from build123d import *

# Parameters (mm, degrees)
SKETCH1_W               = 101.6
SKETCH1_H               = 76.2
BOSS_EXTRUDE1_DEPTH     = 177.8
SHELL1_T                = -5.08
SKETCH2_W               = 2.667
SKETCH2_H               = 2.667
CUT_EXTRUDE1_DEPTH      = 15.24
CUT_EXTRUDE1_DRAFT      = -1
MIRROR1_COPY_1_SKETCH_W = 2.667
MIRROR1_COPY_1_SKETCH_H = 2.667
MIRROR1_COPY_1_DEPTH    = 15.24
MIRROR1_COPY_1_DRAFT    = -1
MIRROR2_COPY_1_SKETCH_W = 2.667
MIRROR2_COPY_1_SKETCH_H = 2.667
MIRROR2_COPY_1_DEPTH    = 15.24
MIRROR2_COPY_1_DRAFT    = -1
MIRROR2_COPY_2_SKETCH_W = 2.667
MIRROR2_COPY_2_SKETCH_H = 2.667
MIRROR2_COPY_2_DEPTH    = 15.24
MIRROR2_COPY_2_DRAFT    = -1
MIRROR3_COPY_1_SKETCH_W = 2.667
MIRROR3_COPY_1_SKETCH_H = 2.667
MIRROR3_COPY_1_DEPTH    = 15.24
MIRROR3_COPY_1_DRAFT    = -1
MIRROR3_COPY_2_SKETCH_W = 2.667
MIRROR3_COPY_2_SKETCH_H = 2.667
MIRROR3_COPY_2_DEPTH    = 15.24
MIRROR3_COPY_2_DRAFT    = -1
MIRROR3_COPY_3_SKETCH_W = 2.667
MIRROR3_COPY_3_SKETCH_H = 2.667
MIRROR3_COPY_3_DEPTH    = 15.24
MIRROR3_COPY_3_DRAFT    = -1
MIRROR3_COPY_4_SKETCH_W = 2.667
MIRROR3_COPY_4_SKETCH_H = 2.667
MIRROR3_COPY_4_DEPTH    = 15.24
MIRROR3_COPY_4_DRAFT    = -1
SKETCH3_W               = 63.5
SKETCH3_H               = 91.44
SKETCH3_W_2             = 58.42
SKETCH3_H_2             = 86.36
EXTRUDE_THIN1_DEPTH     = 12.7
SKETCH4_W               = 25.4
SKETCH4_H               = 91.44
CUT_EXTRUDE_THIN1_DEPTH = 12.7
FILLET1_R               = 2.54


with BuildPart() as part:
    # Sketch1 → Boss-Extrude1 (new body)
    with BuildSketch(Plane(origin=(0, 0, 0), x_dir=(1, 0, 0), z_dir=(0, 1, 0))):
        Rectangle(SKETCH1_W, SKETCH1_H)
    extrude(amount=BOSS_EXTRUDE1_DEPTH)

    # Shell1
    shell1_openings = [part.faces().sort_by_distance(p)[0] for p in [
        (0, 177.8, 0),
        (0, 0, 0),
    ]]
    offset(amount=SHELL1_T, openings=shell1_openings, kind=Kind.INTERSECTION)


with BuildPart() as cut_extrude1_tool:
    # Sketch2 → Cut-Extrude1 (with draft: the straight prism first)
    with BuildSketch(Plane(origin=(0, 177.8, 0), x_dir=(1, 0, 0), z_dir=(0, 1, 0))):
        with Locations((-48.26, 35.56)):
            Rectangle(SKETCH2_W, SKETCH2_H)
    extrude(amount=-CUT_EXTRUDE1_DEPTH)
    # Cut-Extrude1: the draft: its side faces are tilted about the plane it starts from
    cut_extrude1_sides = [cut_extrude1_tool.faces().sort_by_distance(p)[0] for p in [
        (-49.5935, 170.18, -35.56),
        (-48.26, 170.18, -34.2265),
        (-46.9265, 170.18, -35.56),
        (-48.26, 170.18, -36.8935),
    ]]
    draft(cut_extrude1_sides, Plane(origin=(0, 177.8, 0), x_dir=(1, 0, 0), z_dir=(0, 1, 0)), CUT_EXTRUDE1_DRAFT)


with BuildPart() as part_1:
    add(part.part)

    # Cut-Extrude1: cut by cut_extrude1_tool
    add(cut_extrude1_tool.part, mode=Mode.SUBTRACT)


with BuildPart() as mirror1_copy_1_tool:
    # Mirror1 copy 1 sketch → Mirror1 copy 1 (with draft: the straight prism first)
    with BuildSketch(Plane(origin=(0, 177.8, 0), x_dir=(1, 0, 0), z_dir=(0, 1, 0))):
        with Locations((-48.26, -35.56)):
            Rectangle(MIRROR1_COPY_1_SKETCH_W, MIRROR1_COPY_1_SKETCH_H)
    extrude(amount=-MIRROR1_COPY_1_DEPTH)
    # Mirror1 copy 1: the draft: its side faces are tilted about the plane it starts from
    mirror1_copy_1_sides = [mirror1_copy_1_tool.faces().sort_by_distance(p)[0] for p in [
        (-49.5935, 170.18, 35.56),
        (-48.26, 170.18, 34.2265),
        (-46.9265, 170.18, 35.56),
        (-48.26, 170.18, 36.8935),
    ]]
    draft(mirror1_copy_1_sides, Plane(origin=(0, 177.8, 0), x_dir=(1, 0, 0), z_dir=(0, 1, 0)), MIRROR1_COPY_1_DRAFT)


with BuildPart() as part_2:
    add(part_1.part)

    # Mirror1 copy 1: cut by mirror1_copy_1_tool
    add(mirror1_copy_1_tool.part, mode=Mode.SUBTRACT)


with BuildPart() as mirror2_copy_1_tool:
    # Mirror2 copy 1 sketch → Mirror2 copy 1 (with draft: the straight prism first)
    with BuildSketch(Plane(origin=(0, 177.8, 0), x_dir=(-1, 0, 0), z_dir=(0, 1, 0))):
        with Locations((-48.26, -35.56)):
            Rectangle(MIRROR2_COPY_1_SKETCH_W, MIRROR2_COPY_1_SKETCH_H)
    extrude(amount=-MIRROR2_COPY_1_DEPTH)
    # Mirror2 copy 1: the draft: its side faces are tilted about the plane it starts from
    mirror2_copy_1_sides = [mirror2_copy_1_tool.faces().sort_by_distance(p)[0] for p in [
        (49.5935, 170.18, -35.56),
        (48.26, 170.18, -34.2265),
        (46.9265, 170.18, -35.56),
        (48.26, 170.18, -36.8935),
    ]]
    draft(mirror2_copy_1_sides, Plane(origin=(0, 177.8, 0), x_dir=(-1, 0, 0), z_dir=(0, 1, 0)), MIRROR2_COPY_1_DRAFT)


with BuildPart() as part_3:
    add(part_2.part)

    # Mirror2 copy 1: cut by mirror2_copy_1_tool
    add(mirror2_copy_1_tool.part, mode=Mode.SUBTRACT)


with BuildPart() as mirror2_copy_2_tool:
    # Mirror2 copy 2 sketch → Mirror2 copy 2 (with draft: the straight prism first)
    with BuildSketch(Plane(origin=(0, 177.8, 0), x_dir=(-1, 0, 0), z_dir=(0, 1, 0))):
        with Locations((-48.26, 35.56)):
            Rectangle(MIRROR2_COPY_2_SKETCH_W, MIRROR2_COPY_2_SKETCH_H)
    extrude(amount=-MIRROR2_COPY_2_DEPTH)
    # Mirror2 copy 2: the draft: its side faces are tilted about the plane it starts from
    mirror2_copy_2_sides = [mirror2_copy_2_tool.faces().sort_by_distance(p)[0] for p in [
        (49.5935, 170.18, 35.56),
        (48.26, 170.18, 34.2265),
        (46.9265, 170.18, 35.56),
        (48.26, 170.18, 36.8935),
    ]]
    draft(mirror2_copy_2_sides, Plane(origin=(0, 177.8, 0), x_dir=(-1, 0, 0), z_dir=(0, 1, 0)), MIRROR2_COPY_2_DRAFT)


with BuildPart() as part_4:
    add(part_3.part)

    # Mirror2 copy 2: cut by mirror2_copy_2_tool
    add(mirror2_copy_2_tool.part, mode=Mode.SUBTRACT)


with BuildPart() as mirror3_copy_1_tool:
    # Mirror3 copy 1 sketch → Mirror3 copy 1 (with draft: the straight prism first)
    with BuildSketch(Plane.XZ):
        with Locations((-48.26, -35.56)):
            Rectangle(MIRROR3_COPY_1_SKETCH_W, MIRROR3_COPY_1_SKETCH_H)
    extrude(amount=-MIRROR3_COPY_1_DEPTH)
    # Mirror3 copy 1: the draft: its side faces are tilted about the plane it starts from
    mirror3_copy_1_sides = [mirror3_copy_1_tool.faces().sort_by_distance(p)[0] for p in [
        (-49.5935, 7.62, -35.56),
        (-48.26, 7.62, -34.2265),
        (-46.9265, 7.62, -35.56),
        (-48.26, 7.62, -36.8935),
    ]]
    draft(mirror3_copy_1_sides, Plane.XZ, MIRROR3_COPY_1_DRAFT)


with BuildPart() as part_5:
    add(part_4.part)

    # Mirror3 copy 1: cut by mirror3_copy_1_tool
    add(mirror3_copy_1_tool.part, mode=Mode.SUBTRACT)


with BuildPart() as mirror3_copy_2_tool:
    # Mirror3 copy 2 sketch → Mirror3 copy 2 (with draft: the straight prism first)
    with BuildSketch(Plane.XZ):
        with Locations((-48.26, 35.56)):
            Rectangle(MIRROR3_COPY_2_SKETCH_W, MIRROR3_COPY_2_SKETCH_H)
    extrude(amount=-MIRROR3_COPY_2_DEPTH)
    # Mirror3 copy 2: the draft: its side faces are tilted about the plane it starts from
    mirror3_copy_2_sides = [mirror3_copy_2_tool.faces().sort_by_distance(p)[0] for p in [
        (-49.5935, 7.62, 35.56),
        (-48.26, 7.62, 34.2265),
        (-46.9265, 7.62, 35.56),
        (-48.26, 7.62, 36.8935),
    ]]
    draft(mirror3_copy_2_sides, Plane.XZ, MIRROR3_COPY_2_DRAFT)


with BuildPart() as part_6:
    add(part_5.part)

    # Mirror3 copy 2: cut by mirror3_copy_2_tool
    add(mirror3_copy_2_tool.part, mode=Mode.SUBTRACT)


with BuildPart() as mirror3_copy_3_tool:
    # Mirror3 copy 3 sketch → Mirror3 copy 3 (with draft: the straight prism first)
    with BuildSketch(Plane(origin=(0, 0, 0), x_dir=(-1, 0, 0), z_dir=(0, -1, 0))):
        with Locations((-48.26, 35.56)):
            Rectangle(MIRROR3_COPY_3_SKETCH_W, MIRROR3_COPY_3_SKETCH_H)
    extrude(amount=-MIRROR3_COPY_3_DEPTH)
    # Mirror3 copy 3: the draft: its side faces are tilted about the plane it starts from
    mirror3_copy_3_sides = [mirror3_copy_3_tool.faces().sort_by_distance(p)[0] for p in [
        (49.5935, 7.62, -35.56),
        (48.26, 7.62, -34.2265),
        (46.9265, 7.62, -35.56),
        (48.26, 7.62, -36.8935),
    ]]
    draft(mirror3_copy_3_sides, Plane(origin=(0, 0, 0), x_dir=(-1, 0, 0), z_dir=(0, -1, 0)), MIRROR3_COPY_3_DRAFT)


with BuildPart() as part_7:
    add(part_6.part)

    # Mirror3 copy 3: cut by mirror3_copy_3_tool
    add(mirror3_copy_3_tool.part, mode=Mode.SUBTRACT)


with BuildPart() as mirror3_copy_4_tool:
    # Mirror3 copy 4 sketch → Mirror3 copy 4 (with draft: the straight prism first)
    with BuildSketch(Plane(origin=(0, 0, 0), x_dir=(-1, 0, 0), z_dir=(0, -1, 0))):
        with Locations((-48.26, -35.56)):
            Rectangle(MIRROR3_COPY_4_SKETCH_W, MIRROR3_COPY_4_SKETCH_H)
    extrude(amount=-MIRROR3_COPY_4_DEPTH)
    # Mirror3 copy 4: the draft: its side faces are tilted about the plane it starts from
    mirror3_copy_4_sides = [mirror3_copy_4_tool.faces().sort_by_distance(p)[0] for p in [
        (49.5935, 7.62, 35.56),
        (48.26, 7.62, 34.2265),
        (46.9265, 7.62, 35.56),
        (48.26, 7.62, 36.8935),
    ]]
    draft(mirror3_copy_4_sides, Plane(origin=(0, 0, 0), x_dir=(-1, 0, 0), z_dir=(0, -1, 0)), MIRROR3_COPY_4_DRAFT)


with BuildPart() as part_8:
    add(part_7.part)

    # Mirror3 copy 4: cut by mirror3_copy_4_tool
    add(mirror3_copy_4_tool.part, mode=Mode.SUBTRACT)

    # Sketch3 → Extrude-Thin1 (add)
    with BuildSketch(Plane(origin=(0, 0, 33.02), x_dir=(-1, 0, 0), z_dir=(0, 0, -1))):
        with Locations((0, 101.6)):
            Rectangle(SKETCH3_W, SKETCH3_H)
        with Locations((0, 101.6)):
            Rectangle(SKETCH3_W_2, SKETCH3_H_2, mode=Mode.SUBTRACT)
    extrude(amount=EXTRUDE_THIN1_DEPTH)

    # Sketch4 → Cut-Extrude-Thin1 (cut)
    with BuildSketch(Plane(origin=(0, 0, 20.32), x_dir=(-1, 0, 0), z_dir=(0, 0, -1))):
        with Locations((0, 101.6)):
            Rectangle(SKETCH4_W, SKETCH4_H)
    extrude(amount=-CUT_EXTRUDE_THIN1_DEPTH, mode=Mode.SUBTRACT)

    # Fillet1
    fillet1_edges = [part_8.edges().sort_by_distance(p)[0] for p in [
        (50.8, 88.9, 38.1),
        (-50.8, 88.9, 38.1),
        (-50.8, 88.9, -38.1),
        (50.8, 88.9, -38.1),
    ]]
    fillet(fillet1_edges, radius=FILLET1_R)


solid = part_8.part
Input: part model. Units: mm. Frame: model coordinates. A direction names the side the tool comes from. Coordinates: 2 decimals unless noted, no trailing zeros. Loops run counter-clockwise (first coordinate to the right, second up) from the corner with the lowest first, then second, coordinate; pieces in that order, holes last.
(1) Section B-B on z = -30.5. Return the cut outline in (x, y), then the cut area to 3 significant figures.
(2) Section C-C on z = 31. Return the cut outline in (x, y), then the cut area to 3 significant figures.
(3) Set-up query: faces 5 (the face through (22, 147.32, 27)), 6 (the face through (-22, 55.88, 27)), 7 (the face through (21, 144.78, 27)), 8 (the face through (30, 102, 20.32)). Return all of +Z, -Z, +X, -X, +Y, -Y with unobstructed straight access to the full face (end or side cutting, diameter ignored); none if empty.
(4) Material intervals for probe 1 along X at (y, z) = (67, 22); probe 2 along X at (y, z) = (62, -18); probe 3 along Z at (x, y) = (13, 70.5), sorted ascending.
(5) Section A-A on x = 42.5. Return the cut outline in (y, z), then the cut area to 3 significant figures.
(6) Pull-direction query (Z, two-part tool) for faces 1 (the face through (-29.21, 101, 27)), 2 (the face through (45.72, 88, 0)), 3 (the face through (-1, 88, -38.1)), 4 (the face through (50.8, 88, 0)); classes: released by +Z, released by -Z, zero draft, split by the parting line, or undercut.
(7) First-contact query: pin 1 Ø10 at (x, z) = (19.5, 25.5) entering from +Y; pin 2 Ø1.1 at (x, z) = (-48.5, -36) entering from +Y; pin 3 Ø1.1 at (x, z) = (48.5, 35.5) entering from -Y. Flat tips, straight axial feed; report the tip coordinate or a pass-through.
(8) Section D-D on y = 96. Return the cut outline in (x, z).
Data:
1. outline: (-50.8, 0) - (-45.72, 0) - (-45.72, 177.8) - (-50.8, 177.8) - close; (45.72, 0) - (50.8, 0) - (50.8, 177.8) - (45.72, 177.8) - close
1. area: 1,810 mm2
2. outline: (-50.8, 0) - (-45.72, 0) - (-45.72, 177.8) - (-50.8, 177.8) - close; (-31.75, 55.88) - (-12.7, 55.88) - (-12.7, 58.42) - (-29.21, 58.42) - (-29.21, 144.78) - (-12.7, 144.78) - (-12.7, 147.32) - (-31.75, 147.32) - close; (12.7, 55.88) - (31.75, 55.88) - (31.75, 147.32) - (12.7, 147.32) - (12.7, 144.78) - (29.21, 144.78) - (29.21, 58.42) - (12.7, 58.42) - close; (45.72, 0) - (50.8, 0) - (50.8, 177.8) - (45.72, 177.8) - close
2. area: 2,440 mm2
3. face 5: +Y
3. face 6: -Y
3. face 7: none
3. face 8: +Y, -Y
4. probe 1: x = -50.8 to -45.72, -31.75 to -29.21, 29.21 to 31.75, 45.72 to 50.8
4. probe 2: x = -50.8 to -45.72, 45.72 to 50.8
4. probe 3: z = -38.1 to -33.02, 33.02 to 38.1
5. outline: (0, -38.1) - (177.8, -38.1) - (177.8, -33.02) - (0, -33.02) - close; (0, 33.02) - (177.8, 33.02) - (177.8, 38.1) - (0, 38.1) - close
5. area: 1,810 mm2
6. face 1: undercut
6. face 2: undercut
6. face 3: released by -Z
6. face 4: zero draft
7. pin 1: stops at y = 147.32
7. pin 2: stops at y = 162.56
7. pin 3: stops at y = 15.24
8. outline: (-50.8, -35.56) arc R2.54 ccw to (-48.26, -38.1) - (48.26, -38.1) arc R2.54 ccw to (50.8, -35.56) - (50.8, 35.56) arc R2.54 ccw to (48.26, 38.1) - (-48.26, 38.1) arc R2.54 ccw to (-50.8, 35.56) - close; hole (-45.72, -33.02) - (45.72, -33.02) - (45.72, 33.02) - (31.75, 33.02) - (31.75, 20.32) - (29.21, 20.32) - (29.21, 33.02) - (-29.21, 33.02) - (-29.21, 20.32) - (-31.75, 20.32) - (-31.75, 33.02) - (-45.72, 33.02) - close
